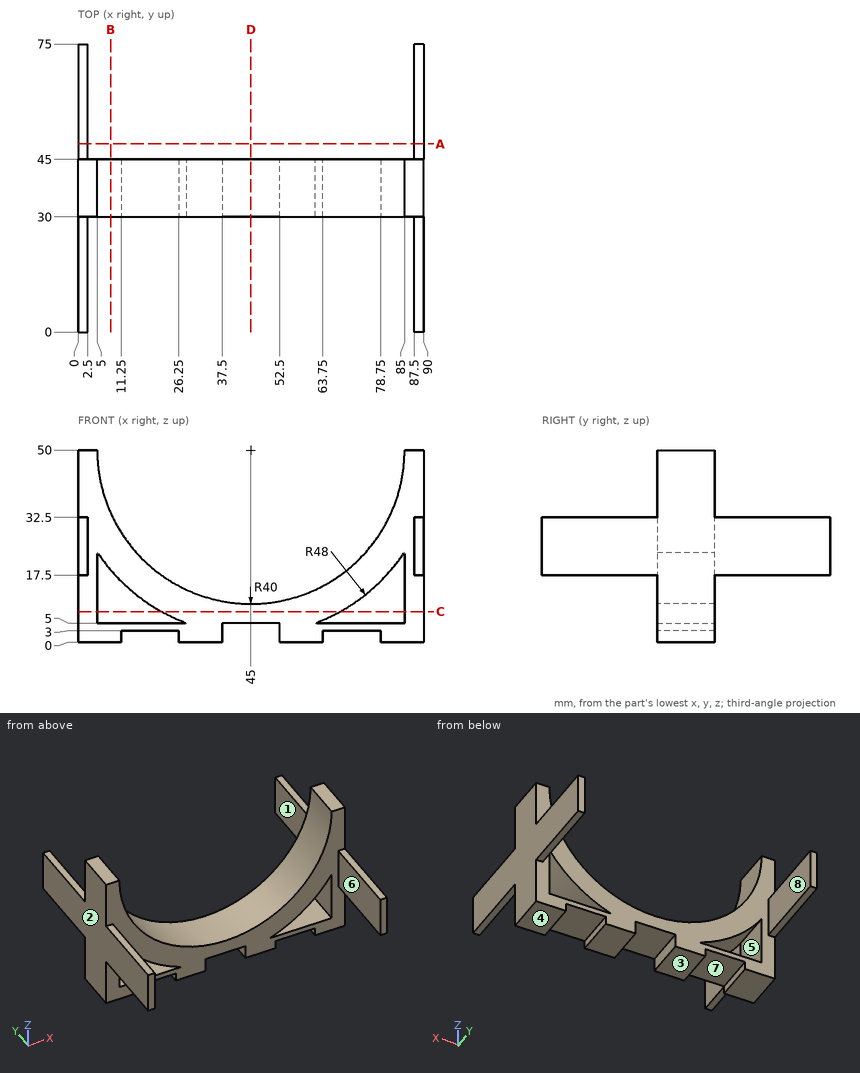
Check sheet for the drawn part. Datum: minimum x, y, z corner. Units: mm. A direction names the side the tool comes from. Round coordinates to 2 decimals unless told otherwise and drop trailing zeros. Write each loop counter-clockwise with the first axis right and the second up, starting at its lowest first coordinate (ties: lowest second). Pieces come first, ordered by that corner, then holes. Notation, with made-up numbers: (78.25, 33) - (83.25, 33) arc R6 ccw to (83.25, 39) - close; hole circle Ø5 at (48.5, 8.25). An arc over 180 degrees is marked (long way). Return JSON: item names as keys, results as strings.
Q1. Draft check along X on the marked faces 1, 2 and 3. Enter one of: released by +X, released by -X, zero draft, split by the parting line, or undercut.
Returned:
{"face 1": "undercut", "face 2": "released by -X", "face 3": "zero draft"}
Q2. Cross-section at D-D (x = 45). Record the boundary of the cut face in (y, z).
Returned:
{"outline": "(30, 5) - (45, 5) - (45, 10) - (30, 10) - close"}
Q3. Cross-section at A-A (y = 49). Record the boundary of the cut face in (x, z).
Returned:
{"outline": "(0, 17.5) - (2.5, 17.5) - (2.5, 32.5) - (0, 32.5) - close; (87.5, 17.5) - (90, 17.5) - (90, 32.5) - (87.5, 32.5) - close"}
Q4. Cross-section at B-B (x = 8.5). Record the boundary of the cut face in (y, z).
Returned:
{"outline": "(30, 0) - (45, 0) - (45, 5) - (30, 5) - close; (30, 18.83) - (45, 18.83) - (45, 33.64) - (30, 33.64) - close"}
Q5. Cross-section at C-C (z = 8). Record the boundary of the cut face in (x, y).
Returned:
{"outline": "(0, 30) - (5, 30) - (5, 45) - (0, 45) - close; (21.76, 30) - (68.24, 30) - (68.24, 45) - (21.76, 45) - close; (85, 30) - (90, 30) - (90, 45) - (85, 45) - close"}
Q6. Depth check by flat-ended pin: P1, Ø15, axis at x = 36, z = 23.5, coming from the -Y side; P2, Ø10, axis at x = 11, z = 39, coming from the +Y side; P3, Ø1.2, axis at x = 2, y = 9.5, coming from the -Z side; P4, Ø1.2, axis at x = 89, y = 65.5, coming from the +Z side. Enter the tip coordinate at first touch or a pass-through.
Returned:
{"P1": "passes through", "P2": "stops at y = 45", "P3": "stops at z = 17.5", "P4": "stops at z = 32.5"}
Q7. Scan lines: L1, parallel to X at y = 22, z = 20.5; L2, parallel to Y at x = 8, z = 23; L3, parallel to X at y = 35, z = 46.5. Record each from-to range of solid material in increasing order. Write a range as from..to.
Returned:
{"L1": "x = 0..2.5, 87.5..90", "L2": "y = 30..45", "L3": "x = 0..5.15, 84.85..90"}
Q8. Access from +Z, -Z, +X, -X, +Y, -Y to the whole of each face (thin tool, end or side, straight path). Record for the marked faces 4, 5, 6, 7 and 8.
Returned:
{"face 4": "-Z, +X, -X, +Y, -Y", "face 5": "+Y, -Y", "face 6": "+Z, -Z, -Y", "face 7": "-Z, +Y, -Y", "face 8": "+Z, -Z, +Y"}
